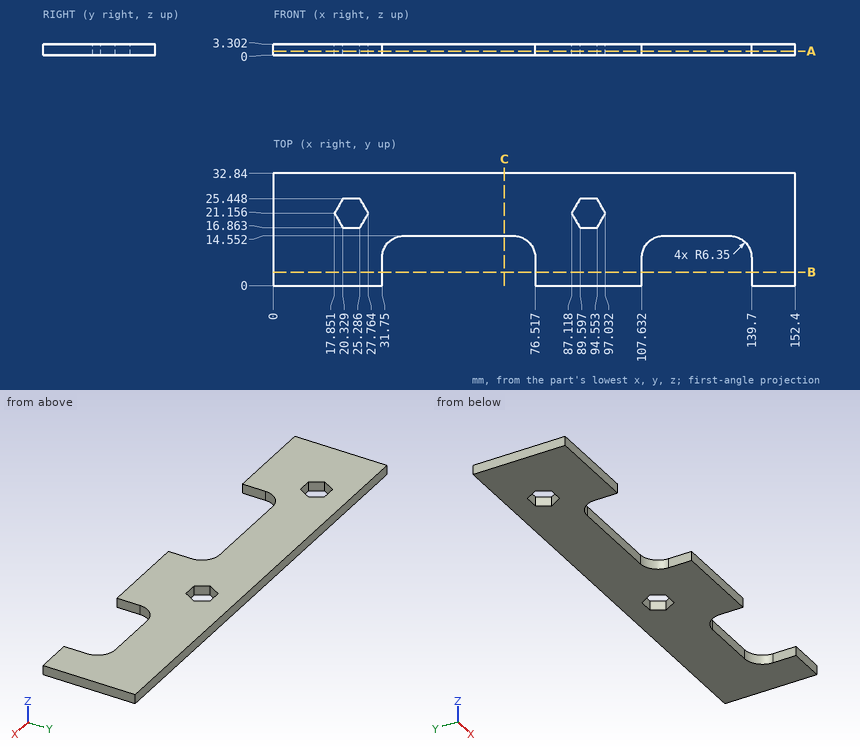
The drawing under review shows one solid part. Ordinate dimensions are in mm from its lowest x, y, z. Round coordinates to 2 decimals unless told otherwise and drop trailing zeros. Write each loop counter-clockwise with the first axis right and the second up, starting at its lowest first coordinate (ties: lowest second). Pieces come first, ordered by that corner, then holes.
(1) Wall thickness on L1, parallel to X at y = 3, z = 2.7; L2, parallel to X at y = 12, z = 2.85 (1 decimal); L3, parallel to Y at x = 120.5, z = 0.45: over which ranges is each line inside the solid? List them lowest first.
(2) We need section B-B on y = 4. Give the boundary of the cut face in (x, z).
(3) We need section A-A on z = 1.25. Give the number of separate pieces and of enclosed holes in the cut face, and give its area (3 significant figures).
(4) We need section C-C on x = 67.5. Give the boundary of the cut face in (y, z).
(5) Insertion check: pin 1 (1 mm diameter, centred on x = 127.5, z = 2, fed in from -Y). The pin has a flat end and moves straight along its axis. Give the tip position at first contact, or say it passes through.
Findings below:
1. L1: x = 0 to 31.75, 76.52 to 107.63, 139.7 to 152.4
1. L2: x = 0 to 33, 75.3 to 108.9, 138.4 to 152.4
1. L3: y = 14.55 to 32.84
2. outline: (0, 0) - (31.75, 0) - (31.75, 3.3) - (0, 3.3) - close; (76.52, 0) - (107.63, 0) - (107.63, 3.3) - (76.52, 3.3) - close; (139.7, 0) - (152.4, 0) - (152.4, 3.3) - (139.7, 3.3) - close
3. separate pieces: 1
3. enclosed holes: 2
3. area: 3,790 mm2
4. outline: (14.55, 0) - (32.84, 0) - (32.84, 3.3) - (14.55, 3.3) - close
5. pin 1: stops at y = 14.55
